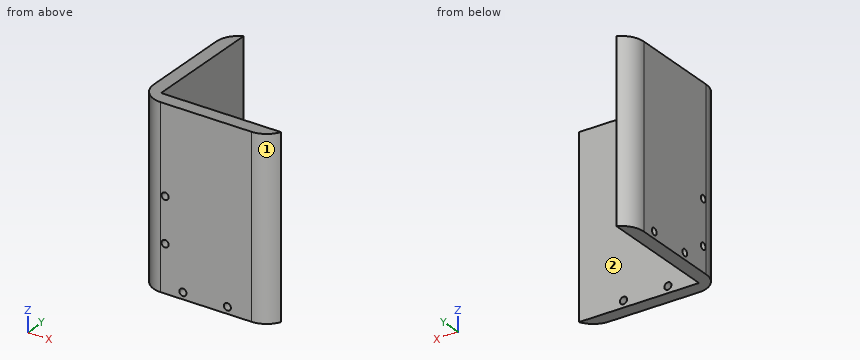
```python
from build123d import *

# Parameters (mm, degrees)
EXTRUDE_1_DEPTH     = 40
FILLET_1_R          = 10
SKETCH_3_R          = 1.55
CUT_EXTRUDE_1_DEPTH = 94.808315196
SKETCH_4_R          = 1.6
CUT_EXTRUDE_2_DEPTH = 91.088845036
SKETCH_5_R          = 1.6
CUT_EXTRUDE_3_DEPTH = 94.808315196


with BuildPart() as part:
    # 草图1 → 凸台-拉伸1 (new, symmetric)
    with BuildSketch(Plane.XY):
        Polygon((0, 0), (0, 60), (6, 60), (6, 6), (60, 6), (60, 0), align=None)
    extrude(amount=EXTRUDE_1_DEPTH, both=True)

    # 圆角1
    # the kernel refuses this fillet: 10 mm, written as the material it takes off along each edge
    with BuildSketch(Plane(origin=(0, 60, 62.912878475), x_dir=(0, -1, 0), z_dir=(0, 0, -1))) as fillet_1_piece_1:
        with BuildLine():
            CenterArc((9.16515139, -10), FILLET_1_R, 90, 66.421821522)
            Line((0, -6), (-0.183303028, -5.92))
            ThreePointArc((-0.183303028, -5.92), (-0.2, -3), (-0.2, 0))
            Line((-0.2, 0), (0, 0.2))
            Line((0, 0.2), (9.16515139, 0.2))
            Line((9.16515139, 0.2), (9.16515139, 0))
        make_face()
    extrude(amount=125.82575695, mode=Mode.SUBTRACT)
    with BuildSketch(Plane(origin=(60, 0, -62.912878475), x_dir=(0, 1, 0), z_dir=(0, 0, 1))) as fillet_1_piece_2:
        with BuildLine():
            CenterArc((10, 9.16515139), FILLET_1_R, 180, 66.421821522)
            Line((0, 9.16515139), (-0.2, 9.16515139))
            Line((-0.2, 9.16515139), (-0.2, 0))
            Line((-0.2, 0), (0, -0.2))
            ThreePointArc((0, -0.2), (3, -0.2), (5.92, -0.183303028))
            Line((5.92, -0.183303028), (6, 0))
        make_face()
    extrude(amount=125.82575695, mode=Mode.SUBTRACT)
    with BuildSketch(Plane(origin=(0, 0, -65), x_dir=(0, 1, 0), z_dir=(0, 0, 1))) as fillet_1_piece_3:
        with BuildLine():
            CenterArc((FILLET_1_R, -FILLET_1_R), FILLET_1_R, 90, 90)
            Line((0, -FILLET_1_R), (-FILLET_1_R * 0.02, -FILLET_1_R))
            Line((-FILLET_1_R * 0.02, -FILLET_1_R), (-FILLET_1_R * 0.02, FILLET_1_R * 0.02))
            Line((-FILLET_1_R * 0.02, FILLET_1_R * 0.02), (FILLET_1_R, FILLET_1_R * 0.02))
            Line((FILLET_1_R, FILLET_1_R * 0.02), (FILLET_1_R, 0))
        make_face()
    extrude(amount=130, mode=Mode.SUBTRACT)

    # 草图3 → 切除-拉伸1 (cut, through all)
    with BuildSketch(Plane.ZY):
        with Locations((-37, 44)):
            Circle(SKETCH_3_R)
        with Locations((-37, 24)):
            Circle(SKETCH_3_R)
        with Locations((-29, 12)):
            Circle(SKETCH_3_R)
        with Locations((-9, 12)):
            Circle(SKETCH_3_R)
    extrude(amount=-CUT_EXTRUDE_1_DEPTH, mode=Mode.SUBTRACT)

    # 草图4 → 切除-拉伸2 (cut, through all)
    with BuildSketch(Plane(origin=(0, 6, 0), x_dir=(1, 0, 0), z_dir=(0, 1, 0))):
        with Locations(Location((12, -1, 0), (0, 0, 270))):
            Circle(SKETCH_4_R)
        with Locations(Location((12, 19, 0), (0, 0, 270))):
            Circle(SKETCH_4_R)
    extrude(amount=-CUT_EXTRUDE_2_DEPTH, mode=Mode.SUBTRACT)

    # 草图5 → 切除-拉伸3 (cut, through all)
    with BuildSketch(Plane.XZ):
        with Locations((20, -37)):
            Circle(SKETCH_5_R)
        with Locations((40, -37)):
            Circle(SKETCH_5_R)
    extrude(amount=-CUT_EXTRUDE_3_DEPTH, mode=Mode.SUBTRACT)


solid = part.part
```
Work out the finished part from the listing and answer in its coordinate system (mm). Face numbers are marked on the shaded views. A direction names the side the tool comes from. Give positions to 0.01 mm unless a question says otherwise; leave off trailing zeros. Order: outer loops, then holes, each group sorted by start corner. A loop starts at its lowest first (then second) coordinate and runs counter-clockwise, first axis right, second up.
1. Section C-C, the plane x = 20 is taken. Determine the outline of the cut face in (y, z), and give its area (3 significant figures).
Result sheet:
outline: (0, -40) - (6, -40) - (6, -38.6) - (0, -38.6) - close; (0, -35.4) - (6, -35.4) - (6, 40) - (0, 40) - close
area: 461 mm2
2. Section D-D, the plane z = -19 is taken. Determine the outline of the cut face in (x, y), and give its area (3 significant figures).
Result sheet:
outline: (0, 10) arc R10 ccw to (10, 0) - (10.4, 0) - (10.4, 6) - (6, 6) - (6, 60) arc R10 ccw to (0, 50.83) - close; (13.6, 0) - (50.83, 0) arc R10 ccw to (60, 6) - (13.6, 6) - close
area: 613 mm2
3. For the marked faces 1 and 2, determine the directions among +Z, -Z, +X, -X, +Y, -Y from which every point of the face is accessible in a straight line to the end or side of a thin tool.
Result sheet:
face 1: +Z, -Z, +X, -Y
face 2: +Z, -Z, +X, +Y
4. Section B-B, the plane y = 12 is taken. Determine the outline of the cut face in (x, z), and give its area (3 significant figures).
Result sheet:
outline: (0, -40) - (6, -40) - (6, -30.55) - (0, -30.55) - close; (0, -27.45) - (6, -27.45) - (6, -10.55) - (0, -10.55) - close; (0, -7.45) - (6, -7.45) - (6, 40) - (0, 40) - close
area: 443 mm2
5. Each of these flat-tipped pins is pushed along its axis until it touches: P1, Ø5, axis at y = 12, z = -29, coming from the -X side; P2, Ø6, axis at x = 29, z = -27, coming from the +Y side; P3, Ø16, axis at y = 22.5, z = -1, coming from the +X side; P4, Ø3, axis at y = 24, z = -37, coming from the -X side. Where does it stop, or does it pass through?
Result sheet:
P1: stops at x = 0
P2: stops at y = 6
P3: stops at x = 6
P4: passes through
6. Section A-A, the plane x = 12 is taken. Determine the outline of the cut face in (y, z).
Result sheet:
outline: (0, -40) - (6, -40) - (6, -20.6) - (0, -20.6) - close; (0, -17.4) - (6, -17.4) - (6, -0.6) - (0, -0.6) - close; (0, 2.6) - (6, 2.6) - (6, 40) - (0, 40) - close
7. Straight lines are drawn through the part: L1, parallel to Y at x = 2, z = -37; L2, parallel to X at y = 24.5, z = -34. For each, find the intervals that lie inside material, in ascending order.
Result sheet:
L1: y = 4 to 22.45, 25.55 to 42.45, 45.55 to 56.83
L2: x = 0 to 6
